Here's how the part is built. I have some questions about the finished solid (model axes, mm). Face numbers are marked on the shaded views. A direction names the side the tool comes from. Coordinates: 2 decimals unless noted, no trailing zeros. Write each loop counter-clockwise with the first axis right and the second up, starting at its lowest first coordinate (ties: lowest second). Pieces come first, ordered by that corner, then holes.
(1) Thinking about a two-plate mould opening in X: for the marked faces 1, 2 and 3, which applies, released by +X, released by -X, zero draft, split by the parting line, or undercut?
(2) Which directions (+Z, -Z, +X, -X, +Y, -Y) give clear straight access to the entire face, cutting with the end or side of a thin tool? Please do the marked faces 4, 5, 6 and 7.
(3) Please list where these lines run through material, in increasing order: probe 1 along Z at (x, y) = (-22, 0) (3 decimals); probe 2 along Y at (x, z) = (-1.5, 7); probe 3 along Y at (x, z) = (-19.65, 6.35).
(4) Imagine slicing it at C-C, the plane z = 6.35. List the corners of the cut face in (x, y) for me, plus the area to 3 significant figures.
(5) Imagine slicing it at A-A, the plane x = 0. List the corners of the cut face in (y, z) for me (3 decimals), plus the area to 3 significant figures.
(6) Imagine slicing it at B-B, the plane z = 10.75. List the corners of the cut face in (x, y) for me.
(7) For pin 1 Ø1.4 at (x, z) = (0.5, 7) entering from -Y; pin 2 Ø4 at (y, z) = (0, 6.35) entering from +X; pin 3 Ø3.5 at (x, z) = (0.5, 7.5) entering from +Y, each with a flat end and sliding along its axis, tell me the tip position at first contact or that it passes through.
Autodesk Inventor part; units mm, degrees
ref_plane "Work Plane1" through (0, 23.7871, 0) normal (0, 1, 0) x (-1, 0, 0)
ref_plane "Work Plane2" through (0, -23.7871, 0) normal (0, -1, 0) x (1, 0, 0)
ref_plane "Work Plane5" through (-23.7871, 0, 0) normal (1, 0, 0) x (0, 1, 0)
sketch "Sketch1" plane through (0, 0, 0) normal (0, 0, 1) x (1, 0, 0)
  circle A0 centre (0, 0) radius 23.7871
  line L0 (3.6808, 6.3754) -> (7.3617, 0)
  line L1 (7.3617, 0) -> (3.6808, -6.3754)
  line L2 (3.6808, -6.3754) -> (-3.6808, -6.3754)
  line L3 (-3.6808, -6.3754) -> (-7.3617, 0)
  line L4 (-7.3617, 0) -> (-3.6808, 6.3754)
  line L5 (-3.6808, 6.3754) -> (3.6808, 6.3754)
  dimension "d0" = 47.5742
  dimension "d2" = 12.7508
extrude "Extrusion1" add sketch "Sketch1" along normal blind 12.7
ref_plane "Work Plane1" through (0, 23.7871, 0) normal (0, 1, 0) x (-1, 0, 0)
sketch "Sketch2" plane through (0, 23.7871, 0) normal (0, 1, 0) x (-1, 0, 0)
  line L0 (23.7871, 12.7) -> (-23.7871, 12.7)
  line L1 (-23.7871, 0) -> (23.7871, 0)
  circle A0 centre (0, 6.35) radius 2.413
  line L2 (0, 0) -> (0, 12.7) construction
  dimension "d5" = 4.826
  dimension "d6" = 6.35
extrude "Extrusion2" cut sketch "Sketch2" against normal blind 5.5563
ref_plane "Work Plane2" through (0, -23.7871, 0) normal (0, -1, 0) x (1, 0, 0)
sketch "Sketch3" plane through (0, -23.7871, 0) normal (0, -1, 0) x (1, 0, 0)
  circle A0 centre (0, 6.35) radius 2.413
  line L0 (23.7871, 12.7) -> (-23.7871, 12.7)
  line L1 (0, 0) -> (0, 12.7) construction
  dimension "d9" = 4.826
  dimension "d10" = 6.35
extrude "Extrusion3" cut sketch "Sketch3" against normal blind 5.5563
ref_plane "Work Plane4" through (23.7871, 0, 0) normal (1, 0, 0) x (0, 1, 0)
ref_plane "Work Plane3" through (7.3617, 0, 0) normal (1, 0, 0) x (0, 0, 1)
sketch "Sketch4" plane through (23.7871, 0, 0) normal (1, 0, 0) x (0, 1, 0)
  line L0 (23.7871, 12.7) -> (-23.7871, 12.7)
  circle A0 centre (0, 6.35) radius 2.413
  line L1 (0, 0) -> (0, 12.7) construction
  dimension "d14" = 4.826
  dimension "d15" = 6.35
extrude "Extrusion4" cut sketch "Sketch4" against normal blind 5.5563
ref_plane "Work Plane5" through (-23.7871, 0, 0) normal (1, 0, 0) x (0, 1, 0)
sketch "Sketch5" plane through (-23.7871, 0, 0) normal (1, 0, 0) x (0, 1, 0)
  line L0 (-23.7871, 0) -> (23.7871, 0)
  circle A0 centre (0, 6.35) radius 2.413
  line L1 (0, 12.6521) -> (0, 0) construction
  dimension "d18" = 4.826
  dimension "d19" = 6.35
extrude "Extrusion5" cut sketch "Sketch5" along normal blind 5.5563
sketch "Sketch6" plane through (0, 0, 12.7) normal (0, 0, 1) x (1, 0, 0)
  line L0 (7.3617, 0) -> (3.6808, -6.3754)
  line L1 (3.6808, -6.3754) -> (-3.6808, -6.3754)
  line L2 (-3.6808, -6.3754) -> (-7.3617, 0)
  line L3 (-7.3617, 0) -> (-3.6808, 6.3754)
  line L4 (-3.6808, 6.3754) -> (3.6808, 6.3754)
  line L5 (3.6808, 6.3754) -> (7.3617, 0)
  circle A0 centre (0, 0) radius 23.7871
  circle A1 centre (0, 0) radius 26.9621
  dimension "d26" = 3.175
extrude "Extrusion6" add sketch "Sketch6" along normal blind 3.175 contours A0 | A1
fillet "Fillet1" radius 0.7937 1 edges at (-23.7871, 0, 12.7)
properties part number "Roller End Cap Drive (3-D Printed)" material "ABS Plastic"
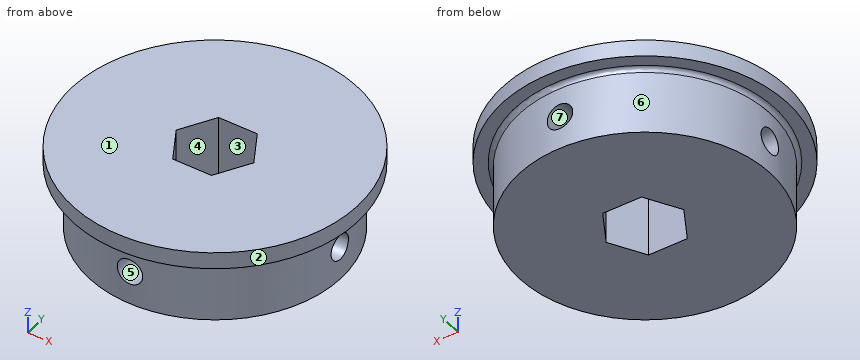
Recorded:
1. face 1: zero draft
1. face 2: split by the parting line
1. face 3: undercut
2. face 4: +Z, -Z
2. face 5: -Y
2. face 6: -Z
2. face 7: +Y
3. probe 1: z = 0 to 3.937, 8.763 to 15.875
3. probe 2: y = -18.23 to -6.38, 6.38 to 18.23
3. probe 3: y = -13.41 to -2.41, 2.41 to 13.41
4. outline: (-23.66, -2.41) arc R23.79 ccw to (-2.41, -23.66) - (-2.41, -18.23) - (2.41, -18.23) - (2.41, -23.66) arc R23.79 ccw to (23.66, -2.41) - (18.23, -2.41) - (18.23, 2.41) - (23.66, 2.41) arc R23.79 ccw to (2.41, 23.66) - (2.41, 18.23) - (-2.41, 18.23) - (-2.41, 23.66) arc R23.79 ccw to (-23.66, 2.41) - (-18.23, 2.41) - (-18.23, -2.41) - close; hole (-7.36, 0) - (-3.68, -6.38) - (3.68, -6.38) - (7.36, 0) - (3.68, 6.38) - (-3.68, 6.38) - close
4. area: 1,530 mm2
5. outline: (-26.962, 12.7) - (-24.581, 12.7) arc R0.794 cw to (-23.787, 11.906) - (-23.787, 8.763) - (-18.231, 8.763) - (-18.231, 3.937) - (-23.787, 3.937) - (-23.787, 0) - (-6.375, 0) - (-6.375, 15.875) - (-26.962, 15.875) - close; (6.375, 0) - (23.787, 0) - (23.787, 3.937) - (18.231, 3.937) - (18.231, 8.763) - (23.787, 8.763) - (23.787, 11.906) arc R0.794 cw to (24.581, 12.7) - (26.962, 12.7) - (26.962, 15.875) - (6.375, 15.875) - close
5. area: 520 mm2
6. outline: circle Ø47.57 at (0, 0); hole (-7.36, 0) - (-3.68, -6.38) - (3.68, -6.38) - (7.36, 0) - (3.68, 6.38) - (-3.68, 6.38) - close
7. pin 1: stops at y = -18.23
7. pin 2: stops at x = 18.23
7. pin 3: stops at y = 23.79
